Verification items for the finished model (mm, model axes). Face numbers are marked on the shaded views. A direction names the side the tool comes from. Coordinates: 2 decimals unless noted, no trailing zeros. Write each loop counter-clockwise with the first axis right and the second up, starting at its lowest first coordinate (ties: lowest second). Pieces come first, ordered by that corner, then holes. Notation, with made-up numbers: (6.5, -20) -> (11.5, -20) arc R16 cw to (11.5, 2) -> close; hole circle Ø7 at (8.5, -5). An arc over 180 degrees is marked (long way). Answer in a Markdown table with one row per item.
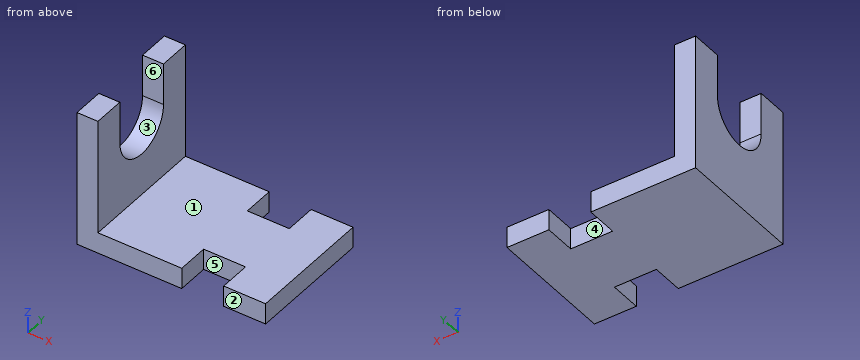
```python
from build123d import *

# Parameters (mm, degrees)
F1_DEPTH = 60
F2_W     = 20
F2_H     = 15
F3_DEPTH = 25
F5_DEPTH = 25


with BuildPart() as f1:
    # F0 (on Front) → F1 (new body)
    with BuildSketch(Plane.XZ):
        Polygon((5, -22.5), (5, 32.5), (-5, 32.5), (-5, -32.5), (5, -32.5), (85, -32.5), (85, -22.5), align=None)
    extrude(amount=-F1_DEPTH)

    # F2 (on face) → F3 (cut)
    with BuildSketch(Plane.XY.offset(-22.5)):
        with Locations((55, 7.5)):
            Rectangle(F2_W, F2_H)
        with Locations((55, 52.5)):
            Rectangle(F2_W, F2_H)
    extrude(amount=-F3_DEPTH, mode=Mode.SUBTRACT)

    # F4 (on face) → F5 (cut)
    with BuildSketch(Plane.YZ.offset(5)):
        with BuildLine():
            Line((15, 32.5), (15, 12.5))
            ThreePointArc((15, 12.5), (30, -2.5), (45, 12.5))
            Line((45, 12.5), (45, 32.5))
            Line((45, 32.5), (15, 32.5))
        make_face()
    extrude(amount=-F5_DEPTH, mode=Mode.SUBTRACT)


solid = f1.part
```
1. Sectioned sample at B-B, the plane y = 53. Record the cut outline in (x, z).
Findings below:
| item | result |
|---|---|
| outline | (-5, -32.5) -> (45, -32.5) -> (45, -22.5) -> (5, -22.5) -> (5, 32.5) -> (-5, 32.5) -> close; (65, -32.5) -> (85, -32.5) -> (85, -22.5) -> (65, -22.5) -> close |
2. Go/stop test with flat-tipped pins: pin 1 (10 mm diameter, centred on x = 59, y = 31, fed in from +Z); pin 2 (11 mm diameter, centred on x = 58, z = -26, fed in from -Y); pin 3 (8 mm diameter, centred on x = 52.5, z = -28, fed in from +Y). Record where each tip stops, or that it passes through.
Findings below:
| item | result |
|---|---|
| pin 1 | stops at z = -22.5 |
| pin 2 | stops at y = 15 |
| pin 3 | stops at y = 45 |
3. Material ranges on probe 1 along X at (y, z) = (56, -28); probe 2 along Y at (x, z) = (4, 17); probe 3 along X at (y, z) = (9.5, 11), recorded low to high. Write a range as from..to.
Findings below:
| item | result |
|---|---|
| probe 1 | x = -5..45, 65..85 |
| probe 2 | y = 0..15, 45..60 |
| probe 3 | x = -5..5 |
4. Sectioned sample at D-D, the plane x = 9. Record the cut outline in (y, z).
Findings below:
| item | result |
|---|---|
| outline | (0, -32.5) -> (60, -32.5) -> (60, -22.5) -> (0, -22.5) -> close |
5. Access from +Z, -Z, +X, -X, +Y, -Y to the whole of each face (thin tool, end or side, straight path). Record for the marked faces 4, 5 and 6.
Findings below:
| item | result |
|---|---|
| face 4 | +Z, -Z, +Y |
| face 5 | +Z, -Z, -Y |
| face 6 | +Z, +X, -X |
6. Sectioned sample at A-A, the plane z = 23. Record the cut outline in (x, y), and give its area (3 significant figures).
Findings below:
| item | result |
|---|---|
| outline | (-5, 0) -> (5, 0) -> (5, 15) -> (-5, 15) -> close; (-5, 45) -> (5, 45) -> (5, 60) -> (-5, 60) -> close |
| area | 300 mm² |
7. Sectioned sample at C-C, the plane y = 30. Record the cut outline in (x, z).
Findings below:
| item | result |
|---|---|
| outline | (-5, -32.5) -> (85, -32.5) -> (85, -22.5) -> (5, -22.5) -> (5, -2.5) -> (-5, -2.5) -> close |
8. Release check for a two-part mould opening along Y. For the marked faces 1, 2 and 3 record: released by +Y, released by -Y, zero draft, split by the parting line, or undercut.
Findings below:
| item | result |
|---|---|
| face 1 | zero draft |
| face 2 | released by -Y |
| face 3 | undercut |
